Design review of the part built by this model. Coordinates are the model's own, in mm. A direction names the side the tool comes from. Give positions to 0.01 mm unless a question says otherwise; leave off trailing zeros. Order: outer loops, then holes, each group sorted by start corner. A loop starts at its lowest first (then second) coordinate and runs counter-clockwise, first axis right, second up. Notation, with made-up numbers: (24.25, 47.5) -> (29.25, 47.5) arc R21 ccw to (29.25, 63.5) -> close; hole circle Ø10 at (13.5, 28). An arc over 180 degrees is marked (long way). One line per item, written item: value. Start each with the question number.
1) Wall thickness on line 1 along Y through (x, z) = (1.1, 1); line 2 along X through (y, z) = (20, 0.3); line 3 along X through (y, z) = (17.5, 0.75): over which ranges is each line inside the solid? List them lowest first. Write a range as from..to.
2) Consider section A-A (z = 1). State the section outline as (x, y) points, plus the area to 3 significant figures.
3) The part is to be moulded in two halves that separate along Z. For faces 4 (the face through (1, 29, 1.3)), 5 (the face through (1, 29, 0.7)), 6 (the face through (30.3, 13.1, 2)), 7 (the face through (16, 2, 1)), say which applies: released by +Z, released by -Z, zero draft, split by the parting line, or undercut.
4) Tool access review of faces 1 (the face through (2, 21.7, 1.5)), 2 (the face through (31, 29, 0.7)), 3 (the face through (36, 17, 1)): name each direction out of +Z, -Z, +X, -X, +Y, -Y from which nothing blocks a thin tool from reaching the whole face with its end or side.
5) Consider section C-C (x = 35.5). State the section outline as (y, z) points, plus the area to 3 significant figures.
6) Consider section D-D (y = 11). State the section outline as (x, z) points, plus the area to 3 significant figures.
7) Consider section B-B (y = 28.5). State the section outline as (x, z) points.
8) For pin 1 (0.5 mm diameter, centred on x = 31, z = 1, fed in from +Y); pin 2 (0.6 mm diameter, centred on y = 28, z = 0.5, fed in from +X), all flat-tipped, find the tip position at first contact; note any pin that passes through.
from build123d import *

# Parameters (mm, degrees)
BOSS_EXTRUDE1_DEPTH     = 2
SKETCH2_R               = 0.36
CUT_EXTRUDE1_DEPTH      = 1
CUT_EXTRUDE1_DEPTH_BACK = 41
BOSS_EXTRUDE2_DEPTH     = 25
BOSS_EXTRUDE3_DEPTH     = 25
CUT_EXTRUDE2_REACH      = 4
SKETCH5_W               = 8
SKETCH5_H               = 25


with BuildPart() as part:
    # Sketch1 → Boss-Extrude1 (new body)
    with BuildSketch(Plane.XY):
        Polygon((2, 17), (2, 2), (30, 2), (30, 17), (40, 17), (40, 0), (0, 0), (0, 17), align=None)
    extrude(amount=BOSS_EXTRUDE1_DEPTH)

    # Sketch2 → Cut-Extrude1 (cut, two sides)
    with BuildSketch(Plane(origin=(40, 0, 0), x_dir=(0, 0, -1), z_dir=(1, 0, 0))) as cut_extrude1_sk:
        with Locations((-1, 9.5)):
            Circle(SKETCH2_R)
    extrude(amount=CUT_EXTRUDE1_DEPTH, mode=Mode.SUBTRACT)
    extrude(cut_extrude1_sk.sketch, amount=-CUT_EXTRUDE1_DEPTH_BACK, mode=Mode.SUBTRACT)

    # Sketch3 → Boss-Extrude2 (add)
    with BuildSketch(Plane(origin=(0, 17, 0), x_dir=(1, 0, 0), z_dir=(0, 1, 0))):
        Polygon((0, -2), (2, -2), (2, -1.3), (0.7, -1.3), (0.7, -0.7), (2, -0.7), (2, 0), (0, 0), align=None)
    extrude(amount=BOSS_EXTRUDE2_DEPTH)

    # Sketch4 → Boss-Extrude3 (add)
    with BuildSketch(Plane(origin=(0, 17, 0), x_dir=(1, 0, 0), z_dir=(0, 1, 0))):
        Polygon((30, -2), (40, -2), (40, 0), (30, 0), (30, -0.7), (31.3, -0.7), (31.3, -1.3), (30, -1.3), align=None)
    extrude(amount=BOSS_EXTRUDE3_DEPTH)

    # Sketch5 → Cut-Extrude2 (cut, up to next)
    with BuildSketch(Plane.XY.offset(2), mode=Mode.PRIVATE) as cut_extrude2_sk1:
        with Locations((36, 29.5)):
            Rectangle(SKETCH5_W, SKETCH5_H)
    cut_extrude2_tool1 = extrude(cut_extrude2_sk1.sketch, amount=-CUT_EXTRUDE2_REACH, mode=Mode.PRIVATE) & part.part
    add(cut_extrude2_tool1.solids().sort_by_distance((36, 29.5, 2))[0], mode=Mode.SUBTRACT)


solid = part.part
Checked values:
1. line 1: y = 0..9.14, 9.86..17
1. line 2: x = 0..2, 30..32
1. line 3: x = 0..0.7, 31.3..32
2. outline: (0, 0) -> (40, 0) -> (40, 9.14) -> (30, 9.14) -> (30, 2) -> (2, 2) -> (2, 9.14) -> (0, 9.14) -> close; (0, 9.86) -> (2, 9.86) -> (2, 17) -> (0.7, 17) -> (0.7, 42) -> (0, 42) -> close; (30, 9.86) -> (40, 9.86) -> (40, 17) -> (32, 17) -> (32, 42) -> (31.3, 42) -> (31.3, 17) -> (30, 17) -> close
2. area: 286 mm^2
3. face 4: undercut
3. face 5: undercut
3. face 6: released by +Z
3. face 7: zero draft
4. face 1: +Z, -Z, +Y
4. face 2: +Y
4. face 3: +Z, -Z, +X, +Y
5. outline: (0, 0) -> (17, 0) -> (17, 2) -> (0, 2) -> close; hole circle Ø0.72 at (9.5, 1)
5. area: 33.6 mm^2
6. outline: (0, 0) -> (2, 0) -> (2, 2) -> (0, 2) -> close; (30, 0) -> (40, 0) -> (40, 2) -> (30, 2) -> close
6. area: 24.0 mm^2
7. outline: (0, 0) -> (2, 0) -> (2, 0.7) -> (0.7, 0.7) -> (0.7, 1.3) -> (2, 1.3) -> (2, 2) -> (0, 2) -> close; (30, 0) -> (32, 0) -> (32, 2) -> (30, 2) -> (30, 1.3) -> (31.3, 1.3) -> (31.3, 0.7) -> (30, 0.7) -> close
8. pin 1: stops at y = 17
8. pin 2: stops at x = 32
